```python
from build123d import *

# Parameters (mm, degrees)
BOSS_EXTRUDE2_DEPTH = 25.4
SKETCH2_R           = 6.35
BOSS_EXTRUDE3_DEPTH = 3.175
SKETCH3_R           = 4.7625
CUT_EXTRUDE1_DEPTH  = 26.19375
SKETCH4_R           = 1.5875
BOSS_EXTRUDE4_DEPTH = 15.875
CUT_EXTRUDE2_START  = -0.254
SKETCH5_R           = 5.55625
SKETCH5_R_2         = 1.5875
CUT_EXTRUDE2_DEPTH  = 0.254
CUT_EXTRUDE4_DEPTH  = 0.127
SKETCH4_4_R         = 0.79375
CUT_EXTRUDE6_DEPTH  = 5.588
CHAMFER1_SIZE       = 0.127


with BuildPart() as part:
    # Sketch1 → Boss-Extrude2 (new body)
    with BuildSketch(Plane(origin=(0, 0, 0), x_dir=(1, 0, 0), z_dir=(0, 1, 0))):
        Polygon((6.35, -9.525), (-6.35, -9.525), (-6.35, 2.630256121), (-2.630256121, 6.35), (2.630256121, 6.35), (6.35, 2.630256121), align=None)
    extrude(amount=-BOSS_EXTRUDE2_DEPTH)

    # Sketch2 → Boss-Extrude3 (add)
    with BuildSketch(Plane.XZ.offset(25.4)):
        with Locations(Location((0, 0, 0), (0, 0, 270))):
            Circle(SKETCH2_R)
    extrude(amount=BOSS_EXTRUDE3_DEPTH)

    # Sketch3 → Cut-Extrude1 (cut)
    with BuildSketch(Plane.XZ.offset(28.575)):
        with Locations(Location((0, 0, 0), (0, 0, 270))):
            Circle(SKETCH3_R)
    extrude(amount=-CUT_EXTRUDE1_DEPTH, mode=Mode.SUBTRACT)

    # Sketch4 → Boss-Extrude4 (add)
    with BuildSketch(Plane.XY.offset(9.525)):
        with Locations((0, -12.7)):
            Circle(SKETCH4_R)
    extrude(amount=BOSS_EXTRUDE4_DEPTH)

    # Sketch5 → Cut-Extrude2 (cut)
    with BuildSketch(Plane.XY.offset(9.525).offset(CUT_EXTRUDE2_START)):
        with Locations((0, -12.7)):
            Circle(SKETCH5_R)
        with Locations((0, -12.7)):
            Circle(SKETCH5_R_2, mode=Mode.SUBTRACT)
    extrude(amount=CUT_EXTRUDE2_DEPTH, mode=Mode.SUBTRACT)

    # Sketch5<4> → Cut-Extrude4 (cut)
    with BuildSketch(Plane.XY.offset(9.525)):
        with BuildLine():
            ThreePointArc((0, 0), (3.287001873, -0.432742006), (6.35, -1.701477372))
            Line((6.35, -1.701477372), (6.35, 0))
            Line((6.35, 0), (0, 0))
        make_face()
        with BuildLine():
            ThreePointArc((-6.35, -1.701477372), (-3.287001873, -0.432742006), (0, 0))
            Line((0, 0), (-6.35, 0))
            Line((-6.35, 0), (-6.35, -1.701477372))
        make_face()
        with BuildLine():
            Line((-6.35, -25.4), (0, -25.4))
            ThreePointArc((0, -25.4), (-3.287001873, -24.967257994), (-6.35, -23.698522628))
            Line((-6.35, -23.698522628), (-6.35, -25.4))
        make_face()
        with BuildLine():
            Line((6.35, -25.4), (6.35, -23.698522628))
            ThreePointArc((6.35, -23.698522628), (3.287001873, -24.967257994), (0, -25.4))
            Line((0, -25.4), (6.35, -25.4))
        make_face()
    extrude(amount=-CUT_EXTRUDE4_DEPTH, mode=Mode.SUBTRACT)

    # Sketch4<4> → Cut-Extrude6 (cut)
    with BuildSketch(Plane.XY.offset(9.525)):
        with Locations((0, -3.175)):
            Circle(SKETCH4_4_R)
    extrude(amount=-CUT_EXTRUDE6_DEPTH, mode=Mode.SUBTRACT)

    # Chamfer1
    chamfer1_edges = [part.edges().sort_by_distance(p)[0] for p in [
        (-1.5875, -12.7, 25.4),
    ]]
    chamfer(chamfer1_edges, length=CHAMFER1_SIZE)


solid = part.part
```
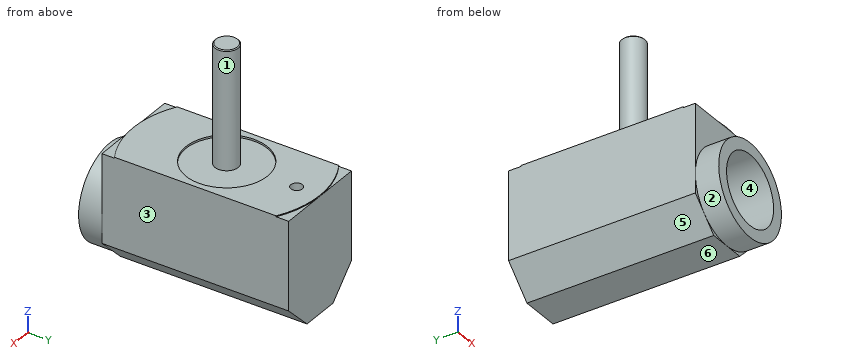
Input: part model. Units: mm. Frame: model coordinates. Face numbers are marked on the shaded views. A direction names the side the tool comes from. Give positions to 0.01 mm unless a question says otherwise; leave off trailing zeros. Order: outer loops, then holes, each group sorted by start corner. A loop starts at its lowest first (then second) coordinate and runs counter-clockwise, first axis right, second up. Notation, with made-up numbers: M 75.25,83.25 L 96.25,83.25 A22 ccw 96.25,117.25 Z; hole C -23.75,0 d4. An arc over 180 degrees is marked long. Return JSON: item names as keys, results as strings.
1) Section query B-B on x = -4. Output: boundary loops of the cut face in (y, z) (3 decimals), and give its area (3 significant figures).
Taken from the geometry:
{"outline": "M -28.575,-4.932 L -25.4,-4.932 L -25.4,-4.98 L 0,-4.98 L 0,9.398 L -0.646,9.398 L -0.646,9.525 L -8.844,9.525 L -8.844,9.271 L -16.556,9.271 L -16.556,9.525 L -24.754,9.525 L -24.754,9.398 L -25.4,9.398 L -25.4,4.932 L -28.575,4.932 L -28.575,2.585 L -2.381,2.585 L -2.381,-2.585 L -28.575,-2.585 Z", "area": "262 mm2"}
2) Line query: L1, parallel to X at y = -23, z = 0; L2, parallel to Y at x = 0, z = 6.95; L3, parallel to Z at x = 0, y = -7.5. Output: solid intervals per line, ascending. Write a range as [from, to].
Taken from the geometry:
{"L1": "x = [-6.35, -4.76], [4.76, 6.35]", "L2": "y = [-25.4, -3.97], [-2.38, 0]", "L3": "z = [-6.35, -4.76], [4.76, 9.27]"}
3) Section query D-D on z = 22.5. Output: boundary loops of the cut face in (x, y) (1 decimal), and give its area (3 significant figures).
Taken from the geometry:
{"outline": "C 0,-12.7 d3.2", "area": "7.92 mm2"}
4) Mould query, pull axis X, two halves, no side actions, for the marked faces 4, 5 and 6. Classes: released by +X, released by -X, zero draft, split by the parting line, or undercut.
Taken from the geometry:
{"face 4": "undercut", "face 5": "released by -X", "face 6": "zero draft"}
5) Access query for the marked faces 1, 2 and 3. Directions: +Z, -Z, +X, -X, +Y, -Y. A direction counts if a zero-diameter tool reaches every point of the face in a straight line with its end or side. Return the directions, or none.
Taken from the geometry:
{"face 1": "+Z", "face 2": "-Y", "face 3": "+Z, -Z, +X, +Y, -Y"}
6) Contact query for flat-ended pins moving along their axis: pin 1 (1.5 mm diameter, centred on x = -3.5, y = -16, fed in from -Z); pin 2 (1.9 mm diameter, centred on x = -3, y = -0.5, fed in from +Z) (3 decimals); pin 3 (1.3 mm diameter, centred on x = 0, y = -3.175, fed in from +Z). Output: stop coordinate, or through.
Taken from the geometry:
{"pin 1": "stops at z = -6.23", "pin 2": "stops at z = 9.525", "pin 3": "stops at z = -4.72"}
